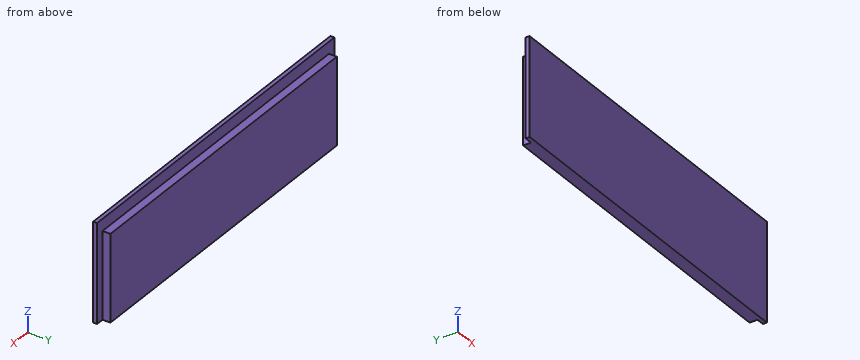
from build123d import *

# Parameters (mm, degrees)
SKETCH026_W             = 526
SKETCH026_H             = 150
PAD010_DEPTH            = 18
SKETCH027_W             = 12
SKETCH027_H             = 150
POCKET016_DEPTH         = 12
SKETCH031_W             = 526
SKETCH031_H             = 18
POCKET019_DEPTH         = 12
BODY009_PLACEMENT_ANGLE = 90


with BuildPart() as part:
    # Sketch026 → Pad010 (new body)
    with BuildSketch(Plane.XY):
        with Locations((0, 75)):
            Rectangle(SKETCH026_W, SKETCH026_H)
    extrude(amount=PAD010_DEPTH)

    # Sketch027 (on Face6 of Pad010) → Pocket016 (cut)
    with BuildSketch(Plane.XY.offset(18)):
        with Locations((-257, 75)):
            Rectangle(SKETCH027_W, SKETCH027_H)
    pocket016 = extrude(amount=-POCKET016_DEPTH, mode=Mode.SUBTRACT)

    # Mirrored007: Pocket016 across Sketch027 V_Axis
    add(pocket016.mirror(Plane(origin=(0, 0, 18), x_dir=(0, 0, 1), z_dir=(1, 0, 0))), mode=Mode.SUBTRACT)

    # Sketch031 (on Face6 of Mirrored007) → Pocket019 (cut)
    with BuildSketch(Plane.XY.offset(18)):
        with Locations((0, 9)):
            Rectangle(SKETCH031_W, SKETCH031_H)
    extrude(amount=-POCKET019_DEPTH, mode=Mode.SUBTRACT)


with BuildPart() as part_1:
    # Body009 placement: moved
    add(part.part.moved(Location((0, 0, 150))).rotate(Axis((0, 0, 150), (-1, 0, 0)), BODY009_PLACEMENT_ANGLE))


solid = part_1.part
Model file for the job. Use its own axes, mm. Coordinates: 2 decimals unless noted, no trailing zeros. Order: outer loops, then holes, each group sorted by start corner. A loop starts at its lowest first (then second) coordinate and runs counter-clockwise, first axis right, second up. Notation, with made-up numbers: (-36, 69.25) -> (6, 69.25) arc R21 ccw to (6, 81.25) -> close; hole circle Ø2 at (13.5, 44.5). An arc over 180 degrees is marked (long way). Return JSON: item names as keys, results as strings. Group by question number.
Item 1: Wall check: line 1 along X through (y, z) = (12, 52); line 2 along Z through (x, y) = (103.5, 8); line 3 along Y through (x, z) = (-7.5, 133). Give the ranges that are in metal, low to high. Write a range as [from, to].
Item 2: Saw through at B-B on z = 120. Write the cut outline in (x, y), then the cut area to 3 significant figures.
Item 3: Saw through at C-C on y = 10.5. Write the cut outline in (x, z), then the cut area to 3 significant figures.
Item 4: Saw through at A-A on x = -190. Write the cut outline in (y, z), then the cut area to 3 significant figures.
Item 5: Flat gauge pins, fed straight in: P1, Ø1, axis at x = 147, y = 14, coming from the +Z side; P2, Ø10, axis at x = -50, y = 2, coming from the -Z side; P3, Ø6, axis at y = 15, z = 79.5, coming from the +X side; P4, Ø4, axis at y = 12, z = 36, coming from the -X side. Where does each tip first touch, or does it go through?
Values found:
{
 "1": {"line 1": "x = [-251, 251]", "line 2": "z = [0, 132]", "line 3": "y = [0, 6]"},
 "2": {"outline": "(-263, 0) -> (263, 0) -> (263, 6) -> (251, 6) -> (251, 18) -> (-251, 18) -> (-251, 6) -> (-263, 6) -> close", "area": "9,180 mm2"},
 "3": {"outline": "(-251, 0) -> (251, 0) -> (251, 132) -> (-251, 132) -> close", "area": "66,300 mm2"},
 "4": {"outline": "(0, 0) -> (18, 0) -> (18, 132) -> (6, 132) -> (6, 150) -> (0, 150) -> close", "area": "2,480 mm2"},
 "5": {"P1": "stops at z = 132", "P2": "stops at z = 0", "P3": "stops at x = 251", "P4": "stops at x = -251"}
}
